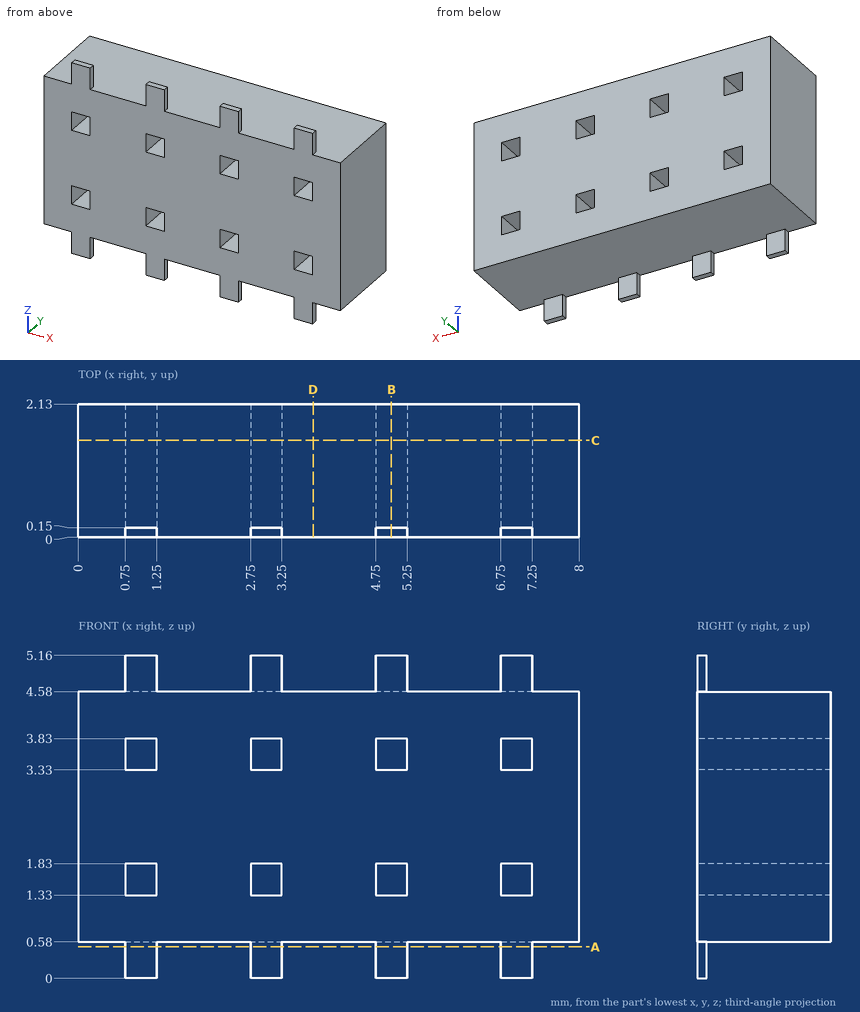
Verification items for this drawing (mm, ordinates from the low corner). Coordinates: 2 decimals unless noted, no trailing zeros. Write each loop counter-clockwise with the first axis right and the second up, starting at its lowest first coordinate (ties: lowest second). Pieces come first, ordered by that corner, then holes. Notation, with made-up numbers: M 15.25,-2 L 68.25,-2 A30 ccw 68.25,35 Z; hole C 58,-6.75 d3. An arc over 180 degrees is marked long. Answer as a JSON object with one key per item and string values.
1. Section check D-D, the plane x = 3.75. Enter the section's corners in (y, z).
Answers below:
{"outline": "M 0,0.58 L 2.13,0.58 L 2.13,4.58 L 0,4.58 Z"}
2. Section check A-A, the plane z = 0.5. Enter the section's corners in (x, y), plus the area to 3 significant figures.
Answers below:
{"outline": "M 0.75,0 L 1.25,0 L 1.25,0.15 L 0.75,0.15 Z; M 2.75,0 L 3.25,0 L 3.25,0.15 L 2.75,0.15 Z; M 4.75,0 L 5.25,0 L 5.25,0.15 L 4.75,0.15 Z; M 6.75,0 L 7.25,0 L 7.25,0.15 L 6.75,0.15 Z", "area": "0.300 mm²"}
3. Section check B-B, the plane x = 5. Enter the section's corners in (y, z), plus the area to 3 significant figures.
Answers below:
{"outline": "M 0,0 L 0.15,0 L 0.15,0.58 L 2.13,0.58 L 2.13,1.33 L 0,1.33 Z; M 0,1.83 L 2.13,1.83 L 2.13,3.33 L 0,3.33 Z; M 0,3.83 L 2.13,3.83 L 2.13,4.58 L 0.15,4.58 L 0.15,5.16 L 0,5.16 Z", "area": "6.56 mm²"}
4. Section check C-C, the plane y = 1.55. Give the number of separate pieces and of enclosed holes in the cut face, plus the area to 3 significant figures.
Answers below:
{"separate pieces": "1", "enclosed holes": "8", "area": "30.0 mm²"}
5. Go/stop test with flat-tipped pins: pin 1 Ø0.6 at (x, y) = (3, 0.5) entering from -Z; pin 2 Ø0.6 at (x, y) = (1, 0.5) entering from +Z. Record where each tip stops, or that it passes through.
Answers below:
{"pin 1": "stops at z = 0.58", "pin 2": "stops at z = 4.58"}
6. Scan lines: L1, parallel to Z at x = 7, y = 1.15; L2, parallel to X at y = 1.6, z = 1.5; L3, parallel to Z at x = 6.5, y = 0.95. Record each from-to range of solid material in increasing order.
Answers below:
{"L1": "z = 0.58 to 1.33, 1.83 to 3.33, 3.83 to 4.58", "L2": "x = 0 to 0.75, 1.25 to 2.75, 3.25 to 4.75, 5.25 to 6.75, 7.25 to 8", "L3": "z = 0.58 to 4.58"}
